Read the model definition and answer for the solid it produces. Units are mm, in the model's axes. Face numbers are marked on the shaded views. A direction names the side the tool comes from. Round coordinates to 2 decimals unless told otherwise and drop trailing zeros. Order: outer loops, then holes, each group sorted by start corner. A loop starts at its lowest first (then second) coordinate and runs counter-clockwise, first axis right, second up. Notation, with made-up numbers: (-39, 29.5) -> (-10, 29.5) arc R17 cw to (-10, 57.5) -> close; hole circle Ø5 at (3, -3.5). An arc over 180 degrees is marked (long way). Answer as a JSON object with one key per item and string values. Group by question number.
Item 1: Section C-C, the plane x = 22 is taken. Write down the section's boundary in (y, z), plus the area to 3 significant figures.
Item 2: Section B-B, the plane x = 4.5 is taken. Write down the section's boundary in (y, z), plus the area to 3 significant figures.
Item 3: The mould has two halves that part along Y. Classify the marked faces 1, 2, 3 and 4: pulls with the +Y half, pulls with the -Y half, needs draft (parallel to the pull), parting line crosses it, or undercut.
Item 4: Given P1, Ø18, axis at x = -5.5, y = 11, coming from the +Z side; P2, Ø11, axis at x = -9, z = -2, coming from the +Y side; P3, Ø5, axis at y = 33, z = 5.5, coming from the +X side, each flat-ended and moving along its own axis, determine where each tip first touches the part or whether it passes through.
Item 5: Section A-A, the plane z = 0 is taken. Write down the section's boundary in (x, y).
Item 6: Section D-D, the plane z = 11.5 is taken. Write down the section's boundary in (x, y), plus the area to 3 significant figures.
Item 7: Consider probe 1 along X at (y, z) = (2.45, 0); probe 2 along Z at (x, y) = (3.5, 5.5); probe 3 along Y at (x, z) = (21, -2.5). Determine where each line is inside the solid, lowest interval first. Write a range as from..to.
Item 8: For the marked faces 5, 6 and 7, determine the directions among +Z, -Z, +X, -X, +Y, -Y from which every point of the face is accessible in a straight line to the end or side of a thin tool.
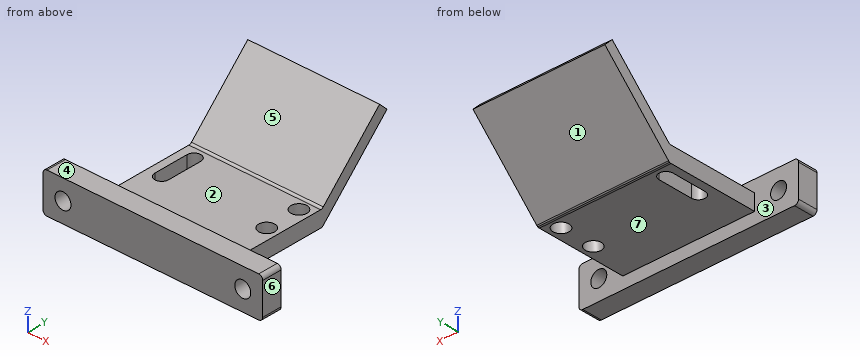
from build123d import *

# Parameters (mm, degrees)
EXTRUDE_2_DEPTH     = 5
SKETCH_4_W          = 33
SKETCH_4_H          = 4
EXTRUDE_3_DEPTH     = 23
EXTRUDE_4_DEPTH     = 33
SKETCH_11_R         = 2
CUT_EXTRUDE_1_DEPTH = 14
CUT_EXTRUDE_2_DEPTH = 33
SKETCH_17_R         = 2
CUT_EXTRUDE_3_DEPTH = 5
SKETCH_19_W         = 37
SKETCH_19_H         = 10
EXTRUDE_5_DEPTH     = 5


with BuildPart() as part:
    # 草图1 → 凸台-拉伸2 (new body)
    with BuildSketch(Plane(origin=(0, 0, 0), x_dir=(1, 0, 0), z_dir=(0, 1, 0))):
        with BuildLine():
            Line((26.533821687, -5), (18.533821687, -5))
            ThreePointArc((18.533821687, -5), (17.826714906, -4.707106781), (17.533821687, -4))
            Line((17.533821687, -4), (17.533821687, -3))
            ThreePointArc((17.533821687, -3), (17.240928468, -2.292893219), (16.533821687, -2))
            Line((16.533821687, -2), (-16.466178313, -2))
            ThreePointArc((-16.466178313, -2), (-17.173285094, -2.292893219), (-17.466178313, -3))
            Line((-17.466178313, -3), (-17.466178313, -4))
            ThreePointArc((-17.466178313, -4), (-17.759071532, -4.707106781), (-18.466178313, -5))
            Line((-18.466178313, -5), (-26.466178313, -5))
            ThreePointArc((-26.466178313, -5), (-27.173285094, -4.707106781), (-27.466178313, -4))
            Line((-27.466178313, -4), (-27.466178313, 4))
            ThreePointArc((-27.466178313, 4), (-27.173285094, 4.707106781), (-26.466178313, 5))
            Line((-26.466178313, 5), (-18.466178313, 5))
            ThreePointArc((-18.466178313, 5), (-17.759071532, 4.707106781), (-17.466178313, 4))
            Line((-17.466178313, 4), (-17.466178313, 3))
            ThreePointArc((-17.466178313, 3), (-17.173285094, 2.292893219), (-16.466178313, 2))
            Line((-16.466178313, 2), (16.533821687, 2))
            ThreePointArc((16.533821687, 2), (17.240928468, 2.292893219), (17.533821687, 3))
            Line((17.533821687, 3), (17.533821687, 4))
            ThreePointArc((17.533821687, 4), (17.826714906, 4.707106781), (18.533821687, 5))
            Line((18.533821687, 5), (26.533821687, 5))
            ThreePointArc((26.533821687, 5), (27.240928468, 4.707106781), (27.533821687, 4))
            Line((27.533821687, 4), (27.533821687, -4))
            ThreePointArc((27.533821687, -4), (27.240928468, -4.707106781), (26.533821687, -5))
        make_face()
    extrude(amount=EXTRUDE_2_DEPTH)

    # 草图4 → 凸台-拉伸3 (add)
    with BuildSketch(Plane(origin=(0, 5, 0), x_dir=(1, 0, 0), z_dir=(0, 1, 0))):
        with Locations((0.033821687, 0)):
            Rectangle(SKETCH_4_W, SKETCH_4_H)
    extrude(amount=EXTRUDE_3_DEPTH)

    # 草图5 → 凸台-拉伸4 (add)
    with BuildSketch(Plane.ZY.offset(16.466178313)):
        with BuildLine():
            ThreePointArc((2, 27.585786438), (2.076120467, 27.96846987), (2.292893219, 28.292893219))
            Line((2.292893219, 28.292893219), (17.54448252, 43.54448252))
            Line((17.54448252, 43.54448252), (15.54448252, 45.54448252))
            Line((15.54448252, 45.54448252), (-1.707106781, 28.292893219))
            ThreePointArc((-1.707106781, 28.292893219), (-1.821797126, 28.155566643), (-1.910179721, 28))
            Line((-1.910179721, 28), (2, 28))
            Line((2, 28), (2, 27.585786438))
        make_face()
    extrude(amount=-EXTRUDE_4_DEPTH)

    # 草图11 → 切除-拉伸1 (cut)
    with BuildSketch(Plane.XY.offset(2)):
        with Locations((13.533821687, 24.952009276)):
            Circle(SKETCH_11_R)
        with Locations((13.533821687, 16.219563599)):
            Circle(SKETCH_11_R)
        with BuildLine():
            Line((-11.034001398, 24.952009276), (-11.034001398, 16.219563599))
            ThreePointArc((-11.034001398, 16.219563599), (-12.750089855, 14.503475142), (-14.466178313, 16.219563599))
            Line((-14.466178313, 16.219563599), (-14.466178313, 24.952009276))
            ThreePointArc((-14.466178313, 24.952009276), (-12.750089855, 26.668097734), (-11.034001398, 24.952009276))
        make_face()
    extrude(amount=-CUT_EXTRUDE_1_DEPTH, mode=Mode.SUBTRACT)

    # 草图16 → 切除-拉伸2 (cut)
    with BuildSketch(Plane.ZY.offset(16.466178313)):
        with BuildLine():
            Line((-1.910179721, 28), (-2, 28))
            Line((-2, 28), (-2, 27.585786438))
            ThreePointArc((-2, 27.585786438), (-1.97728699, 27.797706563), (-1.910179721, 28))
        make_face()
    extrude(amount=-CUT_EXTRUDE_2_DEPTH, mode=Mode.SUBTRACT)

    # 草图17 → 切除-拉伸3 (cut)
    with BuildSketch(Plane(origin=(0, 5, 0), x_dir=(1, 0, 0), z_dir=(0, 1, 0))):
        with Locations((22.533821687, 0)):
            Circle(SKETCH_17_R)
        with Locations((-22.466178313, 0)):
            Circle(SKETCH_17_R)
    extrude(amount=-CUT_EXTRUDE_3_DEPTH, mode=Mode.SUBTRACT)

    # 草图19 → 凸台-拉伸5 (add)
    with BuildSketch(Plane(origin=(0, 5, 0), x_dir=(1, 0, 0), z_dir=(0, 1, 0))):
        with Locations((0.033821687, 0)):
            Rectangle(SKETCH_19_W, SKETCH_19_H)
    extrude(amount=-EXTRUDE_5_DEPTH)


solid = part.part
Values found:
{
 "1": {"outline": "(0, -5) -> (5, -5) -> (5, -1.93) -> (0, -1.93) -> close; (0, 1.93) -> (5, 1.93) -> (5, 5) -> (0, 5) -> close", "area": "30.7 mm2"},
 "2": {"outline": "(0, -5) -> (5, -5) -> (5, -2) -> (27.59, -2) arc R1 ccw to (28.29, -1.71) -> (45.54, 15.54) -> (43.54, 17.54) -> (28.29, 2.29) arc R1 cw to (27.59, 2) -> (5, 2) -> (5, 5) -> (0, 5) -> close", "area": "208 mm2"},
 "3": {"face 1": "pulls with the +Y half", "face 2": "undercut", "face 3": "undercut", "face 4": "needs draft"},
 "4": {"P1": "z = 5", "P2": "y = 33.5", "P3": "x = 16.53"},
 "5": {"outline": "(-27.47, 0) -> (-24.47, 0) -> (-24.47, 5) -> (-27.47, 5) -> close; (-20.47, 0) -> (20.53, 0) -> (20.53, 5) -> (16.53, 5) -> (16.53, 30) -> (-16.47, 30) -> (-16.47, 5) -> (-20.47, 5) -> close; (24.53, 0) -> (27.53, 0) -> (27.53, 5) -> (24.53, 5) -> close; hole (-14.47, 16.22) arc R1.72 ccw to (-11.03, 16.22) -> (-11.03, 24.95) arc R1.72 ccw to (-14.47, 24.95) -> close; hole circle Ø4 at (13.53, 16.22); hole circle Ø4 at (13.53, 24.95)"},
 "6": {"outline": "(-16.47, 37.5) -> (16.53, 37.5) -> (16.53, 41.5) -> (-16.47, 41.5) -> close", "area": "132 mm2"},
 "7": {"probe 1": "-27.47..-24.47, -20.47..20.53, 24.53..27.53", "probe 2": "-2..2", "probe 3": "0..5"},
 "8": {"face 5": "+Z, +X, -X", "face 6": "+Z, -Z, +X, +Y, -Y", "face 7": "-Z, +X, -X, +Y"}
}
